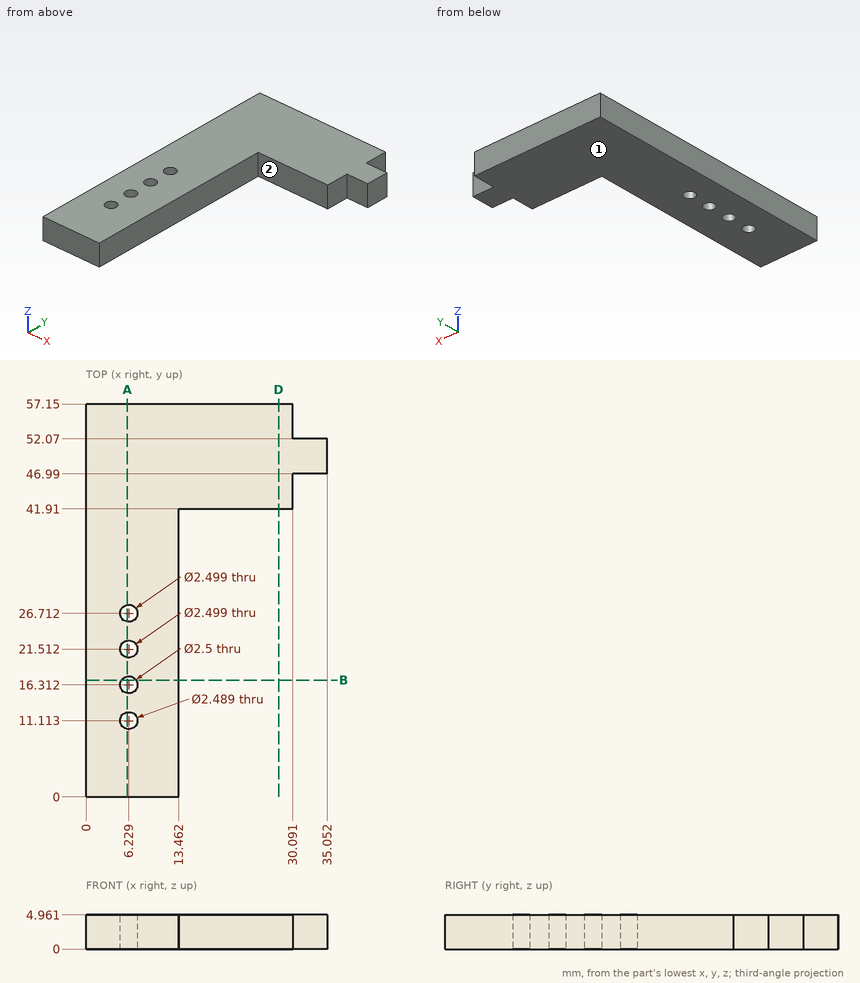
Can you work these out from the drawing? Everything is in mm from the part's minimum corner. A direction names the side the tool comes from. Round coordinates to 2 decimals unless told otherwise and drop trailing zeros. Loops run counter-clockwise (first coordinate to the right, second up) from the corner with the lowest first, then second, coordinate; pieces in that order, holes last. Notation, with made-up numbers: (-29.5, -35) -> (-13.5, -35) arc R6 ccw to (-13.5, -24) -> close; hole circle Ø2 at (32, 40.5). An arc over 180 degrees is marked (long way). Use CSV: the item, a comma, the result in double quotes.
(1) Suppose I cut it at A-A on x = 6. Give the number of separate pieces and of enclosed holes in the cut face, plus the area to 3 significant figures.
Return value:
separate pieces,"5"
enclosed holes,"0"
area,"235 mm²"
(2) Suppose I cut it at B-B on y = 17. Write out the boundary of the cut face in (x, z) (1 decimal).
Return value:
outline,"(0, 0) -> (5.2, 0) -> (5.2, 5) -> (0, 5) -> close; (7.3, 0) -> (13.5, 0) -> (13.5, 5) -> (7.3, 5) -> close"
(3) Suppose I cut it at D-D on x = 28. Write out the boundary of the cut face in (y, z), plus the area to 3 significant figures.
Return value:
outline,"(41.91, 0) -> (57.15, 0) -> (57.15, 4.96) -> (41.91, 4.96) -> close"
area,"75.6 mm²"
(4) For the marked faces 1 and 2, which set-ups out of +Z, -Z, +X, -X, +Y, -Y let a thin tool reach every point of the face, with its end or its side?
Return value:
face 1,"-Z, +X, -X, +Y, -Y"
face 2,"+Z, -Z, +X, -Y"
(5) If I drill on probe 1 along X at (y, z) = (42.5, 1.7); probe 2 along X at (y, z) = (40, 3.8); probe 3 along Y at (x, z) = (33, 1.3), over which ranges is the centre line in solid material (lowest first)? Write a range as [from, to].
Return value:
probe 1,"x = [0, 30.09]"
probe 2,"x = [0, 13.46]"
probe 3,"y = [46.99, 52.07]"
(6) Will these pins go through, and if not, where does the flat tip stop? pin 1 Ø1.5 at (y, z) = (54, 2) entering from +X; pin 2 Ø2 at (x, y) = (6.23, 11.11) entering from -Z; pin 3 Ø1.5 at (x, z) = (25, 1.5) entering from -Y; pin 4 Ø1.5 at (x, z) = (31, 3.5) entering from -Y.
Return value:
pin 1,"stops at x = 30.09"
pin 2,"passes through"
pin 3,"stops at y = 41.91"
pin 4,"stops at y = 46.99"
